Check sheet for the modelled part. Datum: model origin and axes. Units: mm. Face numbers are marked on the shaded views. A direction names the side the tool comes from. Give positions to 0.01 mm unless a question says otherwise; leave off trailing zeros. Write each loop counter-clockwise with the first axis right and the second up, starting at its lowest first coordinate (ties: lowest second). Pieces come first, ordered by that corner, then holes. Notation, with made-up numbers: M 26,-27 L 84,-27 A32 ccw 84,0 Z; hole C -14,41 d11. An arc over 180 degrees is marked long. Write item = value, one per line. Start each with the question number.
1) Set-up check for the marked faces 3, 4 and 5: record each of +Z, -Z, +X, -X, +Y, -Y from which the full face is reachable in a straight line by a thin tool's end or side.
2) Sectioned sample at A-A, the plane z = 14. Record the cut outline in (x, y), then the cut area to 3 significant figures.
3) Draft check along X on the marked faces 1 and 2. Enter one of: pulls with the +X half, pulls with the -X half, needs draft (parallel to the pull), parting line crosses it, or undercut.
4) Gauge pin test, flat ends, axial feed: pin 1 (8 mm diameter, centred on y = -14, z = 18, fed in from +X); pin 2 (12.5 mm diameter, centred on x = 87.5, y = 0.5, fed in from +Z); pin 3 (5.5 mm diameter, centred on y = -3, z = 25.5, fed in from +X). Record the tip position at first contact, or that the pin passes through.
5) Sectioned sample at C-C, the plane y = -2. Count the separate pieces of the cut face and the enclosed holes in it, then the cut area to 3 significant figures.
6) Scan lines: L1, parallel to Y at x = -90, z = 15; L2, parallel to Y at x = 90, z = 7.75; L3, parallel to X at y = -9, z = 16.5. Record each from-to range of solid material in increasing order.
7) Sectioned sample at B-B, the plane x = 17. Record the cut outline in (y, z), then the cut area to 3 significant figures.
from build123d import *

# Parameters (mm, degrees)
F0_R     = 4.2
F1_DEPTH = 10
F2_R     = 12.7
F3_DEPTH = 25
F4_R     = 5
F5_SIZE  = 1


with BuildPart() as f1:
    # F0 (on Top) → F1 (new body)
    with BuildSketch(Plane.XY):
        with BuildLine():
            Line((-70, -10), (-70, 0))
            ThreePointArc((-70, 0), (-104.1421356237, 14.1421356237), (-90, -20))
            Line((-90, -20), (90, -20))
            ThreePointArc((90, -20), (104.1421356237, 14.1421356237), (70, 0))
            Line((70, 0), (70, -10))
            Line((70, -10), (-70, -10))
        make_face()
        with Locations((-90, 0)):
            Circle(F0_R, mode=Mode.SUBTRACT)
        with Locations((90, 0)):
            Circle(F0_R, mode=Mode.SUBTRACT)
    extrude(amount=F1_DEPTH)

    # F2 (on face) → F3 (join)
    with BuildSketch(Plane.XY.offset(10)):
        with BuildLine():
            Line((70, -10), (-70, -10))
            Line((-70, -10), (-70, 0))
            ThreePointArc((-70, 0), (-104.1421356237, 14.1421356237), (-90, -20))
            Line((-90, -20), (90, -20))
            ThreePointArc((90, -20), (104.1421356237, 14.1421356237), (70, 0))
            Line((70, 0), (70, -10))
        make_face()
        with Locations((-90, 0)):
            Circle(F2_R, mode=Mode.SUBTRACT)
        with Locations((90, 0)):
            Circle(F2_R, mode=Mode.SUBTRACT)
    extrude(amount=F3_DEPTH)

    # F4
    f4_edges = [f1.edges().sort_by_distance(p)[0] for p in [
        (-70, -10, 17.5),
        (70, -10, 17.5),
    ]]
    fillet(f4_edges, radius=F4_R)

    # F5
    f5_edges = [f1.edges().sort_by_distance(p)[0] for p in [
        (-70, -2.5, 0),
        (-68.535534, -8.535534, 0),
        (-104.142136, 14.142136, 0),
        (0, -10, 0),
        (0, -20, 0),
        (68.535534, -8.535534, 0),
        (104.142136, 14.142136, 0),
        (70, -2.5, 0),
        (-94.2, 0, 0),
        (85.8, 0, 0),
        (70, -2.5, 35),
        (68.535534, -8.535534, 35),
        (104.142136, 14.142136, 35),
        (0, -10, 35),
        (0, -20, 35),
        (-68.535534, -8.535534, 35),
        (-104.142136, 14.142136, 35),
        (-70, -2.5, 35),
        (-102.7, 0, 35),
        (77.3, 0, 35),
    ]]
    chamfer(f5_edges, length=F5_SIZE)


solid = f1.part
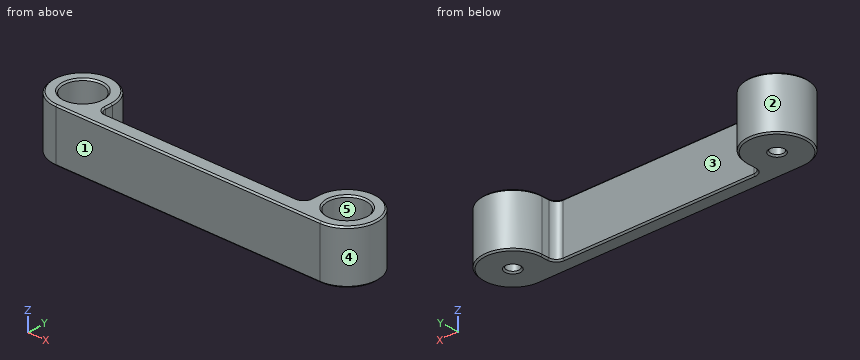
Data:
q1.face_3 = +Z, -Z, +Y
q1.face_4 = +Z, -Z
q1.face_5 = +Z
q2.outline = M -90,-20 L 90,-20 A20 ccw long 70,0 L 70,-5 A5 cw 65,-10 L -65,-10 A5 cw -70,-5 L -70,0 A20 ccw long Z; hole C -90,0 d25.4; hole C 90,0 d25.4
q2.area = 3,080 mm2
q3.face_1 = needs draft
q3.face_2 = undercut
q4.pin_1 = 107.32
q4.pin_2 = 10
q4.pin_3 = 110
q5.separate_pieces = 4
q5.enclosed_holes = 0
q5.area = 1,380 mm2
q6.L1 = -20 to -12.7, 12.7 to 20
q6.L2 = -20 to -4.2, 4.2 to 20
q6.L3 = -107.86 to -98.96, -81.04 to -68, 68 to 81.04, 98.96 to 107.86
q7.outline = M -20,1 L -19,0 L -11,0 L -10,1 L -10,34 L -11,35 L -19,35 L -20,34 Z
q7.area = 348 mm2
